```python
from build123d import *

# Parameters (mm, degrees)
F0_W     = 80
F0_H     = 40
F1_DEPTH = 25
F2_R     = 4
F3_DEPTH = 25
F4_R     = 5
F5_R     = 1


with BuildPart() as f1:
    # F0 (on Top) → F1 (new body)
    with BuildSketch(Plane.XY):
        with Locations((0.1769823041, 3.2334145788)):
            Rectangle(F0_W, F0_H)
        Polygon((40.1769823041, 23.2334145788), (40.1769823041, -16.7665854212), (53.8577880371, 18.2540085112), align=None)
        Polygon((53.8577880371, 60.8211194103), (40.1769823041, 23.2334145788), (53.8577880371, 18.2540085112), (67.5385937702, 55.8417133427), align=None)
    extrude(amount=F1_DEPTH)

    # F2 (on face) → F3 (cut)
    with BuildSketch(Plane(origin=(25.8476953784, 71.0159593971, 0), x_dir=(-0.9396926208, 0.3420201433, 0), z_dir=(0.3420201433, 0.9396926208, 0))):
        with Locations((-37.0871226977, 12.5)):
            Circle(F2_R)
    extrude(amount=-F3_DEPTH, mode=Mode.SUBTRACT)

    # F4
    f4_edges = [f1.edges().sort_by_distance(p)[0] for p in [
        (40.176982, 23.233415, 12.5),
    ]]
    fillet(f4_edges, radius=F4_R)

    # F5
    f5_edges = [f1.edges().sort_by_distance(p)[0] for p in [
        (67.538594, 55.841713, 12.5),
        (60.698191, 58.331416, 0),
        (53.857788, 60.821119, 12.5),
        (60.698191, 58.331416, 25),
    ]]
    fillet(f5_edges, radius=F5_R)


solid = f1.part
```
Design review of the part built by this model. Coordinates are the model's own, in mm. A direction names the side the tool comes from. Give positions to 0.01 mm unless a question says otherwise; leave off trailing zeros. Order: outer loops, then holes, each group sorted by start corner. A loop starts at its lowest first (then second) coordinate and runs counter-clockwise, first axis right, second up. Notation, with made-up numbers: (28, 36.25) - (43, 36.25) arc R20 ccw to (43, 41.25) - close; hole circle Ø11 at (9, 42). An arc over 180 degrees is marked (long way). Use a Markdown table: item, result. Add a question column.
(1) Clearance check with flat-ended pins moving along their axes: P1, Ø3, axis at y = 31, z = 11, coming from the -X side; P2, Ø3, axis at y = 45, z = 22, coming from the +X side; P3, Ø1, axis at y = 36.5, z = 10.5, coming from the -X side. State where each tip first meets the part, or that it passes through.
(2) Mouldability with a two-part tool opening along X and no side actions: class faces 1 (the face through (60.5, 58.1, 24.7)), 2 (the face through (39.509, 24.113, 12.675)), 3 (the face through (-2, 23.233, 12)), 4 (the face through (52.898, 48.055, 13.701)) as +X half, -X half, draft (parallel to the pull), parting line (faces both ways), or undercut.
(3) Add section A-A on z = 19. Give the boundary of the cut face in (x, y).
(4) Machinability: for faces 5 (the face through (13, 14, 25)), 6 (the face through (52.2, 34.82, 12.56)), which of the approach directions +Z, -Z, +X, -X, +Y, -Y give a long, thin tool a straight path to every point of the face, cutting with its end or side? Answer none if there is none.
(5) Wall thickness on probe 1 along Y at (x, z) = (-3, 17.75); probe 2 along Z at (x, y) = (53, 43.5); probe 3 along X at (y, z) = (28.5, 20): over which ranges is each line inside the solid? List them lowest first. Write a range as [from, to].
(6) Add section B-B on y = 7. Give the boundary of the cut face in (x, z), then the cut area to 3 significant figures.
(7) Add section C-C on x = -5. Give the boundary of the cut face in (y, z).
Report:
| question | item | result |
|---|---|---|
| 1 | P1 | stops at x = 42.46 |
| 1 | P2 | stops at x = 64.14 |
| 1 | P3 | stops at x = 44.82 |
| 2 | face 1 | +X half |
| 2 | face 2 | -X half |
| 2 | face 3 | draft |
| 2 | face 4 | undercut |
| 3 | outline | (-39.82, -16.77) - (40.18, -16.77) - (53.86, 18.25) - (67.2, 54.9) arc R1 ccw to (66.6, 56.18) - (54.8, 60.48) arc R1 ccw to (53.52, 59.88) - (41.37, 26.52) arc R5 cw to (36.68, 23.23) - (-39.82, 23.23) - close |
| 4 | face 5 | +Z, +X, -X, +Y, -Y |
| 4 | face 6 | none |
| 5 | probe 1 | y = [-16.77, 23.23] |
| 5 | probe 2 | z = [0, 9.13], [15.87, 25] |
| 5 | probe 3 | x = [42.09, 57.59] |
| 6 | outline | (-39.82, 0) - (49.46, 0) - (49.46, 25) - (-39.82, 25) - close |
| 6 | area | 2,230 mm² |
| 7 | outline | (-16.77, 0) - (23.23, 0) - (23.23, 25) - (-16.77, 25) - close |
